Geometry: final body of the model. Coordinates: model frame, mm. A direction names the side the tool comes from. Coordinates: 2 decimals unless noted, no trailing zeros. Order: outer loops, then holes, each group sorted by start corner. A loop starts at its lowest first (then second) coordinate and runs counter-clockwise, first axis right, second up. Notation, with made-up numbers: (-11, 3) -> (30, 3) arc R17 ccw to (30, 23) -> close; hole circle Ø3 at (6, 42). An arc over 180 degrees is marked (long way). Use CSV: the item, a comma, the result in double quotes. Start each with the question number.
from build123d import *

# Parameters (mm, degrees)
F1_DEPTH      = 40
F1_DEPTH_BACK = 11
F4_DEPTH      = 35
F4_DEPTH_BACK = 27.9057510197
F5_T1_DEPTH   = 14.5743949702
F5_T3_DEPTH   = 14.6258479297


# Not quite as in the source:
# - a fillet or chamfer that OpenCascade refuses, or shapes differently, is made with other operations: its cross-section is extruded or revolved along the edge and cut away or added


with BuildPart() as f1:
    # F0 (on Front) → F1 (new body, two sides)
    with BuildSketch(Plane.XZ) as f1_sk:
        with BuildLine():
            Line((-19.5, 15.5), (-61.5, 15.5))
            ThreePointArc((-61.5, 15.5), (-62.0026261084, 7.75), (-61.5, 0))
            ThreePointArc((-61.5, 0), (-0.0044648026, 1.8801470046), (61.5, 0.319182139))
            ThreePointArc((61.5, 0.319182139), (62.0026261084, 8.069182139), (61.5, 15.819182139))
            Line((61.5, 15.819182139), (19.5, 15.819182139))
            ThreePointArc((19.5, 15.819182139), (0.0077989053, 14.7066639823), (-19.5, 15.5))
        make_face()
    extrude(amount=F1_DEPTH)
    extrude(f1_sk.sketch, amount=-F1_DEPTH_BACK)

    # F3 (on face) → F4 (cut, two sides)
    with BuildSketch(Plane(origin=(0, -8.7376098383, -10.4130779155), x_dir=(1, 0, 0), z_dir=(0, -0.6427876097, -0.7660444431))) as f4_sk:
        with BuildLine():
            Line((41.9965417924, 21), (0, 20.9813332936))
            Line((0, 20.9813332936), (-42.034011751, 20.9813332936))
            ThreePointArc((-42.034011751, 20.9813332936), (-55.2445439017, 11.0585633209), (-64.5, -2.6277822851))
            Line((-64.5, -2.6277822851), (-64.5, -10.626510717))
            Line((-64.5, -10.626510717), (-64.5, -28.2158330083))
            Line((-64.5, -28.2158330083), (0, -28.2158330083))
            Line((0, -28.2158330083), (64.5, -28.2158330083))
            Line((64.5, -28.2158330083), (64.5, -12.4673116952))
            Line((64.5, -12.4673116952), (64.5, -2.6264255467))
            ThreePointArc((64.5, -2.6264255467), (55.2297238243, 11.0740614176), (41.9965417924, 21))
        make_face()
        with BuildLine():
            Line((64.5, 1.9813332936), (64.5, 22.9813332936))
            Line((64.5, 22.9813332936), (64.5, 52.9813332936))
            Line((64.5, 52.9813332936), (-64.5, 52.9813332936))
            Line((-64.5, 52.9813332936), (-64.5, 22.9813332936))
            Line((-64.5, 22.9813332936), (-64.5, 1.9813332936))
            ThreePointArc((-64.5, 1.9813332936), (-55.1354627813, 14.1946752549), (-42.5, 22.9813332936))
            Line((-42.5, 22.9813332936), (42.5, 22.9813332936))
            ThreePointArc((42.5, 22.9813332936), (55.1354627813, 14.1946752549), (64.5, 1.9813332936))
        make_face()
    extrude(amount=-F4_DEPTH, mode=Mode.SUBTRACT)
    extrude(f4_sk.sketch, amount=F4_DEPTH_BACK, mode=Mode.SUBTRACT)

    # F5: fillet of radius 2 on 2 edges, made by hand

    # F5_s2 → F5_t1 (cut)
    with BuildSketch(Plane.XZ.offset(-1.1764499881)):
        with BuildLine():
            ThreePointArc((61.7168527659, 2.2201536136), (61.0312003552, 0.8993903708), (59.6231546265, 0.4177868017))
            ThreePointArc((59.6231546265, 0.4177868017), (60.5615983725, 0.3688853121), (61.5, 0.319182139))
            ThreePointArc((61.5, 0.319182139), (61.6160042169, 1.2688034371), (61.7168527659, 2.2201536136))
        make_face()
    extrude(amount=F5_T1_DEPTH, mode=Mode.SUBTRACT)

    # F5_s4 → F5_t3 (cut)
    with BuildSketch(Plane.XZ.offset(-0.9347638385)):
        with BuildLine():
            ThreePointArc((-59.6137615285, 0.1089088503), (-61.0283512081, 0.5866856233), (-61.7178391039, 1.9110500173))
            ThreePointArc((-61.7178391039, 1.9110500173), (-61.6165778825, 0.9546520415), (-61.5, 0))
            ThreePointArc((-61.5, 0), (-60.5569041472, 0.0548594049), (-59.6137615285, 0.1089088503))
        make_face()
    extrude(amount=F5_T3_DEPTH, mode=Mode.SUBTRACT)


solid = f1.part
(1) Section A-A (x = 49). Return loops of the section in (y, z), then the cut area to 3 significant figures.
(2) Access query for faces 5 (the face through (53.5, -9.29, 8.85)), 6 (the face through (-61.994, 1.686, 8.743)), 7 (the face through (-44, -14, 15.5)). Directions: +Z, -Z, +X, -X, +Y, -Y. A direction counts if a zero-diameter tool reaches every point of the face in a straight line with its end or side. Return the directions, or none.
(3) Line query: line 1 (X direction, y = -8.5, z = 10.5); line 2 (X direction, y = -4, z = 7.75); line 3 (Z direction, x = -39, y = -16.5). Output: solid intervals per line, ascending. Write a range as from..to.
(4) First-contact query: pin 1 (8 mm diameter, centred on y = -16, z = 2, fed in from +X); pin 2 (3 mm diameter, centred on x = -6.5, y = -22, fed in from -Z); pin 3 (1.5 mm diameter, centred on x = 37.5, y = -23, fed in from -Z). Flat tips, straight axial feed; report the tip coordinate or a pass-through.
(5) Mould query, pull axis X, two halves, no side actions, for faces 1 (the face through (62, 1.9, 8.5)), 2 (the face through (0.28, -16.01, 14.71)), 3 (the face through (-53.232, -9.705, 8.747)), 4 (the face through (-0.59, -23.05, 8.28)). Classes: pulls with the +X half, pulls with the -X half, needs draft (parallel to the pull), parting line crosses it, or undercut.
(6) Section B-B (x = -6.5). Return loops of the section in (y, z).
Check sheet entries:
1,outline,"(-24.28, 0.92) -> (-20.91, 0.92) -> (-8.41, 15.82) -> (-11.77, 15.82) -> close"
1,area,"50.2 mm^2"
2,face 5,"-Z, +Y"
2,face 6,"-X, +Y, -Y"
2,face 7,"+Z, -X, +Y, -Y"
3,line 1,"x = -56.09..-53.01, 53.01..56.09"
3,line 2,"x = -60.6..-57.89, 57.89..60.6"
3,line 3,"z = 12.98..15.5"
4,pin 1,"stops at x = 59.29"
4,pin 2,"stops at z = 4.63"
4,pin 3,"stops at z = 4.36"
5,face 1,"pulls with the +X half"
5,face 2,"undercut"
5,face 3,"undercut"
5,face 4,"needs draft"
6,outline,"(-28.45, 1.84) -> (-25.84, 1.84) -> (-15, 14.76) -> (-17.62, 14.76) -> close"
